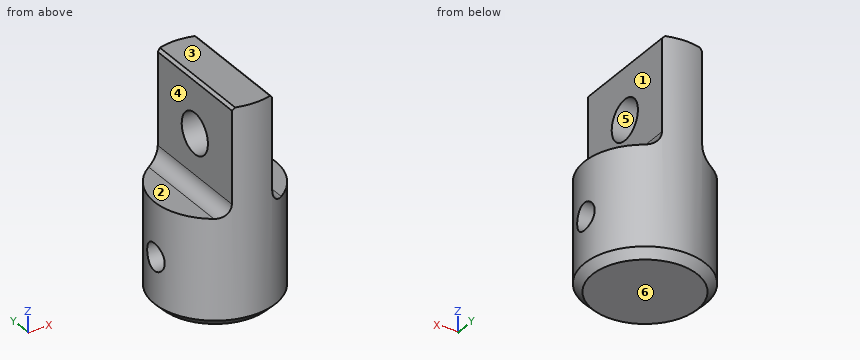
```python
from build123d import *

# Parameters (mm, degrees)
SKETCH_1_R               = 22.5
EXTRUDE_1_DEPTH          = 80
CUT_EXTRUDE_START        = -40
CUT_EXTRUDE_1_DEPTH      = 40
FILLET_1_R               = 5
SKETCH_3_R               = 7.5
CUT_EXTRUDE_2_DEPTH      = 89.352985385
CHAMFER_2_SIZE           = 1
CHAMFER_3_SIZE           = 3
CUT_EXTRUDE_3_DEPTH      = 87.095876934
CUT_EXTRUDE_3_DEPTH_BACK = 87.095876934
SKETCH_4_R               = 5


with BuildPart() as part:
    # Эскиз1 → Бобышка-Вытянуть1 (new body)
    with BuildSketch(Plane.XY):
        Circle(SKETCH_1_R)
    extrude(amount=EXTRUDE_1_DEPTH)

    # Эскиз2 → Вырез-Вытянуть1 (cut)
    with BuildSketch(Plane.XY.offset(80).offset(CUT_EXTRUDE_START)):
        with BuildLine():
            Line((7.5, 21.213203436), (7.5, -21.213203436))
            ThreePointArc((7.5, -21.213203436), (22.5, 0), (7.5, 21.213203436))
        make_face()
        with BuildLine():
            Line((-7.5, 21.213203436), (-7.5, -21.213203436))
            ThreePointArc((-7.5, -21.213203436), (-22.5, 0), (-7.5, 21.213203436))
        make_face()
    extrude(amount=CUT_EXTRUDE_1_DEPTH, mode=Mode.SUBTRACT)

    # Скругление1
    fillet_1_edges = [part.edges().sort_by_distance(p)[0] for p in [
        (-7.5, 0, 40),
        (7.5, 0, 40),
    ]]
    fillet(fillet_1_edges, radius=FILLET_1_R)

    # Эскиз3 → Вырез-Вытянуть2 (cut, through all)
    with BuildSketch(Plane(origin=(7.5, 0, 0), x_dir=(0, 0, -1), z_dir=(1, 0, 0))):
        with Locations((-60, 0)):
            Circle(SKETCH_3_R)
    extrude(amount=-CUT_EXTRUDE_2_DEPTH, mode=Mode.SUBTRACT)

    # Фаска2
    chamfer_2_edges = [part.edges().sort_by_distance(p)[0] for p in [
        (-7.5, 0, 80),
        (7.5, 0, 80),
    ]]
    chamfer(chamfer_2_edges, length=CHAMFER_2_SIZE)

    # Фаска3
    chamfer_3_edges = [part.edges().sort_by_distance(p)[0] for p in [
        (-22.5, 0, 0),
    ]]
    chamfer(chamfer_3_edges, length=CHAMFER_3_SIZE)

    # Эскиз4 → Вырез-Вытянуть3 (cut, two sides: drawn at the far end of the back side and taken through both)
    with BuildSketch(Plane(origin=(0, 0, 0), x_dir=(0, 0, -1), z_dir=(1, 0, 0)).offset(-CUT_EXTRUDE_3_DEPTH_BACK)):
        with Locations((-20, 0)):
            Circle(SKETCH_4_R)
    extrude(amount=CUT_EXTRUDE_3_DEPTH + CUT_EXTRUDE_3_DEPTH_BACK, mode=Mode.SUBTRACT)


solid = part.part
```
Geometry check sheet. Reference: the model listing, model coordinates, mm. Face numbers are marked on the shaded views. A direction names the side the tool comes from. Give positions to 0.01 mm unless a question says otherwise; leave off trailing zeros. Loops run counter-clockwise (first coordinate to the right, second up) from the corner with the lowest first, then second, coordinate; pieces in that order, holes last. Notation, with made-up numbers: M 20,50.5 L 54,50.5 A17 cw 54,61.5 Z; hole C -19,21 d4. An arc over 180 degrees is marked long. Answer as CSV lines item,"result".
Item 1: Access from +Z, -Z, +X, -X, +Y, -Y to the whole of each face (thin tool, end or side, straight path). Record for the marked faces 1, 2 and 3.
Values:
face 1,"+Z, +X, +Y, -Y"
face 2,"+Z, -X, +Y, -Y"
face 3,"+Z, +X, -X, +Y, -Y"
Item 2: Cross-section at D-D on z = 26.5. Record the cut outline in (x, y), and give its area (3 significant figures).
Values:
outline,"C 0,0 d45"
area,"1,590 mm²"
Item 3: Cross-section at C-C on x = 0. Record the cut outline in (y, z), and give its area (3 significant figures).
Values:
outline,"M -22.5,3 L -19.5,0 L 19.5,0 L 22.5,3 L 22.5,80 L -22.5,80 Z; hole C 0,60 d15; hole C 0,20 d10"
area,"3,340 mm²"
Item 4: Cross-section at B-B on z = 60. Record the cut outline in (x, y).
Values:
outline,"M -7.5,-21.21 A22.5 ccw 7.5,-21.21 L 7.5,-7.5 L -7.5,-7.5 Z; M -7.5,7.5 L 7.5,7.5 L 7.5,21.21 A22.5 ccw -7.5,21.21 Z"
Item 5: Material ranges on line 1 (Y direction, x = -0.5, z = 60); line 2 (Y direction, x = 0, z = 5); line 3 (Z direction, x = -9, y = -2.5), recorded low to high.
Values:
line 1,"y = -22.49 to -7.5, 7.5 to 22.49"
line 2,"y = -22.5 to 22.5"
line 3,"z = 0 to 15.67, 24.33 to 41.43"
Item 6: Depth check by flat-ended pin: P1, Ø3, axis at y = 4.5, z = 49.5, coming from the +X side; P2, Ø8, axis at x = -17, y = -9, coming from the +Z side; P3, Ø1.5, axis at x = 4.5, z = 24, coming from the +Y side. Enter the tip coordinate at first touch or a pass-through.
Values:
P1,"stops at x = 7.5"
P2,"stops at z = 40"
P3,"stops at y = 22.19"
Item 7: Release check for a two-part mould opening along Z. For the marked faces 4, 5 and 6 record: pulls with the +Z half, pulls with the -Z half, needs draft (parallel to the pull), parting line crosses it, or undercut.
Values:
face 4,"needs draft"
face 5,"undercut"
face 6,"pulls with the -Z half"
Item 8: Cross-section at A-A on y = 0. Record the cut outline in (x, z), and give its area (3 significant figures).
Values:
outline,"M -22.5,3 L -19.5,0 L 19.5,0 L 22.5,3 L 22.5,15 L -22.5,15 Z; M -22.5,25 L 22.5,25 L 22.5,40 L 12.5,40 A5 cw 7.5,45 L 7.5,52.5 L -7.5,52.5 L -7.5,45 A5 cw -12.5,40 L -22.5,40 Z; M -7.5,67.5 L 7.5,67.5 L 7.5,79 L 6.5,80 L -6.5,80 L -7.5,79 Z"
area,"1,730 mm²"
